from build123d import *

# Parameters (mm, degrees)
F0_R     = 1.5875
F0_R_2   = 2.3749
F0_R_3   = 2.38125
F1_DEPTH = 1.89738


with BuildPart() as f1:
    # F0 (on Front) → F1 (new body)
    with BuildSketch(Plane.XZ):
        with BuildLine():
            ThreePointArc((3.515968, 12.368282), (1.81795, 13.053273), (0.001909, 13.286659))
            Line((0.001909, 13.286659), (-15.875, 13.286659))
            ThreePointArc((-15.875, 13.286659), (-18.120064, 12.356723), (-19.05, 10.111659))
            Line((-19.05, 10.111659), (-19.05, 6.175039))
            ThreePointArc((-19.05, 6.175039), (-17.702166, 3.578486), (-14.803016, 3.186482))
            ThreePointArc((-14.803016, 3.186482), (-8.330226, 3.072112), (-3.557411, -1.30171))
            ThreePointArc((-3.557411, -1.30171), (0.227554, -3.583606), (4.331067, -1.942206))
            ThreePointArc((4.331067, -1.942206), (4.929075, -0.959296), (5.137535, 0.172193))
            Line((5.137535, 0.172193), (5.137535, 9.599262))
            ThreePointArc((5.137535, 9.599262), (4.702314, 11.203705), (3.515968, 12.368282))
        make_face()
        Circle(F0_R, mode=Mode.SUBTRACT)
        with Locations((-13.345532, 8.142169)):
            Circle(F0_R_2, mode=Mode.SUBTRACT)
        with Locations((0, 8.142169)):
            Circle(F0_R_3, mode=Mode.SUBTRACT)
    extrude(amount=F1_DEPTH)


solid = f1.part
The listing builds one solid part. Answer for the finished solid, in the listing's coordinates (mm). Round coordinates to 2 decimals unless told otherwise and drop trailing zeros. Write each loop counter-clockwise with the first axis right and the second up, starting at its lowest first coordinate (ties: lowest second). Pieces come first, ordered by that corner, then holes. Notation, with made-up numbers: M -38,12.25 L -11,12.25 A16 cw -11,23.25 Z; hole C 53,51 d4. An arc over 180 degrees is marked long. Write each question's results on one line, items separated by ' | '. Start each with the question number.
(1) Determine the mould class of faces 1 (the cylindrical face through (-13.86, -0.935, 5.824)), 2 (the flat face through (-4, -1.897, 7)), 3 (the cylindrical face through (4.714, -0.935, 11.183)) for opening direction Z: +Z half, -Z half, draft (parallel to the pull), parting line (faces both ways), or undercut.
(2) The part is cut by section C-C, the plane z = 11.5. Write down the section's boundary in (x, y), and give its area (3 significant figures).
(3) The part is cut by section B-B, the plane x = -12.25. Write down the section's boundary in (y, z), and give its area (3 significant figures).
(4) Find the intervals of material crossed by line 1 (Z direction, x = 0, y = -1.35); line 2 (X direction, y = -1.5, z = -1.25); line 3 (X direction, y = -0.35, z = -0.5), in increasing order.
(5) The part is cut by section D-D, the plane x = -16.5. Write down the section's boundary in (y, z), and give its area (3 significant figures).
(6) The part is cut by section A-A, the plane y = -0.95. Give the number of separate pieces and of enclosed holes in the cut face, and give its area (3 significant figures).
Worked answers:
1) face 1: undercut | face 2: draft | face 3: +Z half
2) outline: M -18.73,-1.9 L 4.51,-1.9 L 4.51,0 L -18.73,0 Z | area: 44.1 mm²
3) outline: M -1.9,3.71 L 0,3.71 L 0,6.04 L -1.9,6.04 Z; M -1.9,10.25 L 0,10.25 L 0,13.29 L -1.9,13.29 Z | area: 10.2 mm²
4) line 1: z = -3.56 to -1.59, 1.59 to 5.76, 10.52 to 13.29 | line 2: x = -3.58 to -0.98, 0.98 to 4.8 | line 3: x = -4.01 to -1.51, 1.51 to 5.07
5) outline: M -1.9,3.06 L 0,3.06 L 0,13.22 L -1.9,13.22 Z | area: 19.3 mm²
6) separate pieces: 1 | enclosed holes: 3 | area: 252 mm²
